Can you work these out from the model? Positions are in its coordinate system, mm. Round coordinates to 2 decimals unless told otherwise and drop trailing zeros. Order: outer loops, then holes, each group sorted by start corner. A loop starts at its lowest first (then second) coordinate and runs counter-clockwise, first axis right, second up. Notation, with made-up numbers: (24.5, 44) -> (63.5, 44) arc R28 ccw to (63.5, 70) -> close; hole circle Ø5 at (-22.5, 39). An arc over 180 degrees is marked (long way). Use a Markdown table: item, result. Add a question column.
Q1. I need wall thicknesses on line 1 along X through (y, z) = (0.75, -19); line 2 along X through (y, z) = (1.75, -20.5); line 3 along Y through (x, z) = (21.5, -1.75). Which ranges of each line are inside material? Lowest first, please. Write a range as [from, to].
Q2. If we section it at A-A on z = -19: List the corners of the cut face in (x, y) for me.
Q3. If we section it at D-D on x = 52: List the corners of the cut face in (y, z) for me, plus the area to 3 significant figures.
Q4. We'd pull the mould along Z, two halves only. Please class faces 1 (the face through (53.115, 1.479, -20.216)), 2 (the face through (33, 1, -22.494)), 3 (the face through (16.902, 7.93, 1.984)): +Z half, -Z half, draft (parallel to the pull), parting line (faces both ways), or undercut.
Q5. If we section it at B-B on x = 31: List the corners of the cut face in (y, z) for me.
Q6. I'm going to push flat-ended pins straight in: pin 1 Ø4 at (x, z) = (31, 0) entering from +Y; pin 2 Ø2 at (x, y) = (14.5, 6.5) entering from -Z; pin 3 Ø1.5 at (x, y) = (35, 3.5) entering from +Z. Where does each tip first touch, or does it pass through?
Q7. If we section it at C-C on y = 1.5: List the corners of the cut face in (x, z) for me.
```python
from build123d import *

# Parameters (mm, degrees)
SKETCH1_R            = 1.65
MAIN_BODY_DEPTH      = 3
SKETCH2_R            = 2.5
CONNECTING_ROD_DEPTH = 10
FILLET1_R            = 2


with BuildPart() as part:
    # Sketch1 → Main Body (new body)
    with BuildSketch(Plane(origin=(0, 0, 0), x_dir=(1, 0, 0), z_dir=(0, 1, 0))):
        with BuildLine():
            Line((9, -4), (9, 22.493705841))
            Line((9, 22.493705841), (21, 22.493705841))
            Line((21, 22.493705841), (57, 22.493705841))
            Line((57, 22.493705841), (57, 21))
            Line((57, 21), (57, 16))
            ThreePointArc((57, 16), (42.206880906, 10.507775049), (36, -4))
            Line((36, -4), (9, -4))
        make_face()
        with Locations(Location((31, 19, 0), (0, 0, 270))):
            Circle(SKETCH1_R, mode=Mode.SUBTRACT)
        with Locations(Location((40, 19, 0), (0, 0, 270))):
            Circle(SKETCH1_R, mode=Mode.SUBTRACT)
        with Locations(Location((52, 19, 0), (0, 0, 270))):
            Circle(SKETCH1_R, mode=Mode.SUBTRACT)
        with Locations(Location((31, 0, 0), (0, 0, 270))):
            Circle(SKETCH1_R, mode=Mode.SUBTRACT)
    extrude(amount=MAIN_BODY_DEPTH)

    # Sketch2 → Connecting Rod (add)
    with BuildSketch(Plane(origin=(0, 3, 0), x_dir=(1, 0, 0), z_dir=(0, 1, 0))):
        with Locations(Location((15.380746581, 0, 0), (0, 0, 90))):
            Circle(SKETCH2_R)
    extrude(amount=CONNECTING_ROD_DEPTH)

    # Fillet1
    fillet1_edges = [part.edges().sort_by_distance(p)[0] for p in [
        (57, 1.5, -22.493705841),
        (57, 1.5, -16),
        (36, 1.5, 4),
        (9, 1.5, 4),
        (9, 1.5, -22.493705841),
    ]]
    fillet(fillet1_edges, radius=FILLET1_R)


solid = part.part
```
Answer below:
| question | item | result |
|---|---|---|
| 1 | line 1 | [9, 29.35], [32.65, 38.35], [41.65, 50.35], [53.65, 57] |
| 1 | line 2 | [9, 30.31], [31.69, 39.31], [40.69, 51.31], [52.69, 57] |
| 1 | line 3 | [0, 3] |
| 2 | outline | (9, 0) -> (29.35, 0) -> (29.35, 3) -> (9, 3) -> close; (32.65, 0) -> (38.35, 0) -> (38.35, 3) -> (32.65, 3) -> close; (41.65, 0) -> (50.35, 0) -> (50.35, 3) -> (41.65, 3) -> close; (53.65, 0) -> (57, 0) -> (57, 3) -> (53.65, 3) -> close |
| 3 | outline | (0, -22.49) -> (3, -22.49) -> (3, -20.65) -> (0, -20.65) -> close; (0, -17.35) -> (3, -17.35) -> (3, -15.62) -> (0, -15.62) -> close |
| 3 | area | 10.7 mm² |
| 4 | face 1 | undercut |
| 4 | face 2 | -Z half |
| 4 | face 3 | parting line |
| 5 | outline | (0, -22.49) -> (3, -22.49) -> (3, -20.65) -> (0, -20.65) -> close; (0, -17.35) -> (3, -17.35) -> (3, -1.65) -> (0, -1.65) -> close; (0, 1.65) -> (3, 1.65) -> (3, 4) -> (0, 4) -> close |
| 6 | pin 1 | y = 3 |
| 6 | pin 2 | z = -2.5 |
| 6 | pin 3 | z = 3.97 |
| 7 | outline | (9, -20.49) arc R2 ccw to (11, -22.49) -> (55, -22.49) arc R2 ccw to (57, -20.49) -> (57, -18) arc R2 ccw to (55.09, -16) arc R20 cw to (36.08, 2.18) arc R2 ccw to (34.09, 4) -> (11, 4) arc R2 ccw to (9, 2) -> close; hole circle Ø3.3 at (31, -19); hole circle Ø3.3 at (31, 0); hole circle Ø3.3 at (40, -19); hole circle Ø3.3 at (52, -19) |
